```python
from build123d import *

# Parameters (mm, degrees)
F0_W      = 72.093084
F0_H      = 61.611962
F1_DEPTH  = 5
F3_W      = 67.553579
F3_H      = 40.44101
F4_DEPTH  = 1
F5_W      = 60.304923
F5_H      = 36.530194
F6_DEPTH  = 2.5
F7_W      = 34.983285
F7_H      = 9.354526
F8_DEPTH  = 5.1
F9_W      = 2.782536
F9_H      = 23.125896
F10_DEPTH = 4.3


with BuildPart() as f1:
    # F0 (on Front) → F1 (new body)
    with BuildSketch(Plane.XZ):
        with Locations((36.046542, 30.805981)):
            Rectangle(F0_W, F0_H)
    extrude(amount=F1_DEPTH)

    # F3 (on face) → F4 (cut)
    with BuildSketch(Plane.XZ.offset(5)):
        with Locations((36.171169, 37.390875)):
            Rectangle(F3_W, F3_H)
    extrude(amount=-F4_DEPTH, mode=Mode.SUBTRACT)

    # F5 (on face) → F6 (join)
    with BuildSketch(Plane(origin=(0, 0, 0), x_dir=(-1, 0, 0), z_dir=(0, 1, 0))):
        with Locations((-34.995176, 29.835877)):
            Rectangle(F5_W, F5_H)
    extrude(amount=F6_DEPTH)

    # F7 (on face) → F8 (cut)
    with BuildSketch(Plane(origin=(0, 2.5, 0), x_dir=(-1, 0, 0), z_dir=(0, 1, 0))):
        with Locations((-34.057569, 28.984568)):
            Rectangle(F7_W, F7_H)
    extrude(amount=-F8_DEPTH, mode=Mode.SUBTRACT)

    # F9 (on face) → F10 (cut)
    with BuildSketch(Plane.YZ.offset(72.093084)):
        with Locations((-2.496595, 16.498187)):
            Rectangle(F9_W, F9_H)
    extrude(amount=-F10_DEPTH, mode=Mode.SUBTRACT)


solid = f1.part
```
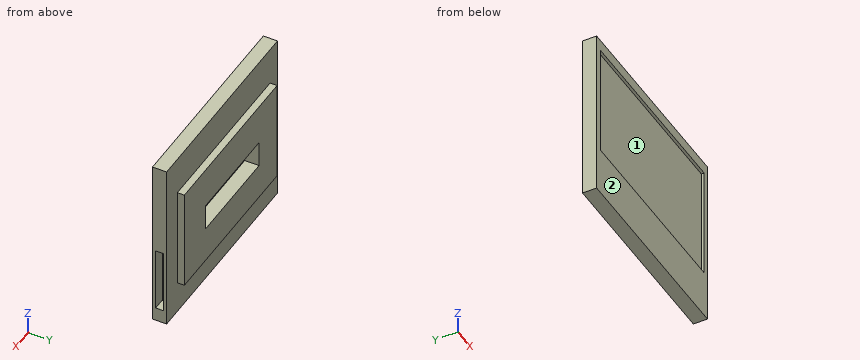
Geometry: final body of the model. Coordinates: model frame, mm. Face numbers are marked on the shaded views. Coordinates: 2 decimals unless noted, no trailing zeros. Order: outer loops, then holes, each group sorted by start corner. A loop starts at its lowest first (then second) coordinate and runs counter-clockwise, first axis right, second up. Notation, with made-up numbers: (76.25, -19) - (91.25, -19) arc R22 ccw to (91.25, 6) - close; hole circle Ø8 at (-3, 78.25). An arc over 180 degrees is marked (long way). Return JSON: item names as keys, results as strings. Group by question number.
1. Pin query (flat end, axial travel): pin 1 (0.8 mm diameter, centred on x = 29, y = 0.5, fed in from +Z); pin 2 (2 mm diameter, centred on x = 42, z = 28.5, fed in from +Y); pin 3 (3.5 mm diameter, centred on x = 69.5, z = 13.5, fed in from +Y). Return the tip coordinate at first contact, or that it passes through.
2. Cut plane D-D (z = 15). Output: boundary loops of the cut face in (x, y).
3. Cut plane A-A (x = 22). Output: boundary loops of the cut face in (y, z), plus the area to 3 significant figures.
4. Material intervals for line 1 along Z through (x, y) = (25.5, 0.5); line 2 along X through (y, z) = (0.25, 31.5); line 3 along Z through (x, y) = (39, -1), sorted ascending. Write a range as [from, to].
5. Cut plane C-C (z = 37). Output: boundary loops of the cut face in (x, y).
6. Cut plane B-B (y = 1.5). Output: boundary loops of the cut face in (x, z).
7. Pull-direction query (X, two-part tool) for the marked faces 1 and 2; classes: pulls with the +X half, pulls with the -X half, needs draft (parallel to the pull), parting line crosses it, or undercut.
Resolved:
{
 "1": {"pin 1": "stops at z = 48.1", "pin 2": "stops at y = -2.6", "pin 3": "stops at y = 0"},
 "2": {"outline": "(0, -5) - (72.09, -5) - (72.09, -3.89) - (67.79, -3.89) - (67.79, -1.11) - (72.09, -1.11) - (72.09, 0) - (65.15, 0) - (65.15, 2.5) - (4.84, 2.5) - (4.84, 0) - (0, 0) - close"},
 "3": {"outline": "(-5, 0) - (0, 0) - (0, 11.57) - (2.5, 11.57) - (2.5, 24.31) - (-2.6, 24.31) - (-2.6, 33.66) - (2.5, 33.66) - (2.5, 48.1) - (0, 48.1) - (0, 61.61) - (-5, 61.61) - (-5, 57.61) - (-4, 57.61) - (-4, 17.17) - (-5, 17.17) - close", "area": "311 mm²"},
 "4": {"line 1": "z = [11.57, 24.31], [33.66, 48.1]", "line 2": "x = [4.84, 16.57], [51.55, 65.15]", "line 3": "z = [0, 24.31], [33.66, 61.61]"},
 "5": {"outline": "(0, -5) - (2.39, -5) - (2.39, -4) - (69.95, -4) - (69.95, -5) - (72.09, -5) - (72.09, 0) - (65.15, 0) - (65.15, 2.5) - (4.84, 2.5) - (4.84, 0) - (0, 0) - close"},
 "6": {"outline": "(4.84, 11.57) - (65.15, 11.57) - (65.15, 48.1) - (4.84, 48.1) - close; hole (16.57, 24.31) - (51.55, 24.31) - (51.55, 33.66) - (16.57, 33.66) - close"},
 "7": {"face 1": "undercut", "face 2": "needs draft"}
}
